Can you work these out from the model? Positions are in its coordinate system, mm. Coordinates: 2 decimals unless noted, no trailing zeros. Loops run counter-clockwise (first coordinate to the right, second up) from the corner with the lowest first, then second, coordinate; pieces in that order, holes last. Notation, with made-up numbers: (-23, 45) -> (11, 45) arc R27 cw to (11, 69) -> close; hole circle Ø6 at (-18.75, 54.25). An arc over 180 degrees is marked (long way). Use one line per item in the form item = value. Start each with the question number.
(1) I need wall thicknesses on line 1 (Z direction, x = -78.5, y = -2.2); line 2 (Z direction, x = -51, y = -2.05); line 3 (X direction, y = -1.1, z = -20). Which ranges of each line are inside material? Lowest first, please. Write a range as [from, to].
(2) Imagine slicing it at B-B (x = -54.5). List the corners of the cut face in (y, z) for me.
(3) Imagine slicing it at A-A (z = -20). List the corners of the cut face in (x, y) for me.
(4) Imagine slicing it at C-C (y = -1.3). List the corners of the cut face in (x, z) for me.
```python
from build123d import *

# Parameters (mm, degrees)
F0_W     = 100
F0_H     = 40
F1_DEPTH = 3
F3_D     = 3
F7_DEPTH = 25
F8_R     = 10


with BuildPart() as f1:
    # F0 (on Front) → F1 (new body)
    with BuildSketch(Plane.XZ):
        with Locations((-50, -20)):
            Rectangle(F0_W, F0_H)
    extrude(amount=F1_DEPTH)

    # F3 (through all)
    with Locations(Plane(origin=(0, 0, 0), x_dir=(1, 0, 0), z_dir=(0, 1, 0))):
        with Locations((-51, 20), (-75, 20)):
            Hole(F3_D / 2)

    # F6 (on face) → F7 (cut)
    with BuildSketch(Plane.XZ.offset(3)):
        with BuildLine():
            ThreePointArc((-80, -27.5), (-82.5, -30), (-80, -32.5))
            Line((-80, -32.5), (-40, -32.5))
            ThreePointArc((-40, -32.5), (-37.5, -30), (-40, -27.5))
            Line((-40, -27.5), (-80, -27.5))
        make_face()
    extrude(amount=-F7_DEPTH, mode=Mode.SUBTRACT)

    # F8
    f8_edges = [f1.edges().sort_by_distance(p)[0] for p in [
        (-100, -1.5, -40),
        (0, -1.5, -40),
    ]]
    fillet(f8_edges, radius=F8_R)

    # F9: F1 across plane


with BuildPart() as f1_1:
    add(f1.part)
    add(f1.part.mirror(Plane.XY))


solid = f1_1.part
```
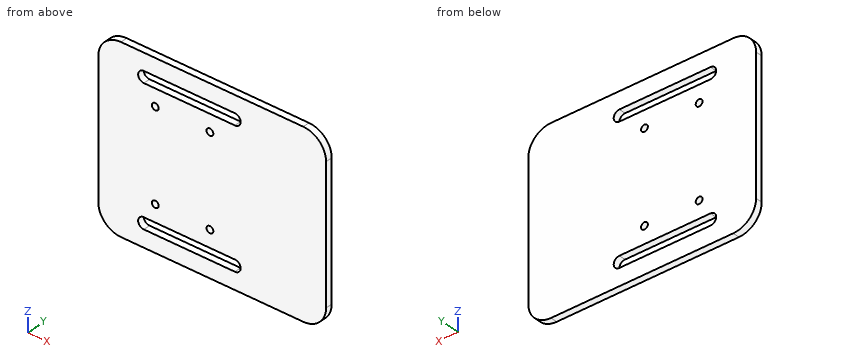
Worked out:
q1.line_1 = [-40, -32.5], [-27.5, 27.5], [32.5, 40]
q1.line_2 = [-40, -32.5], [-27.5, -21.5], [-18.5, 18.5], [21.5, 27.5], [32.5, 40]
q1.line_3 = [-100, -76.5], [-73.5, -52.5], [-49.5, 0]
q2.outline = (-3, -40) -> (0, -40) -> (0, -32.5) -> (-3, -32.5) -> close; (-3, -27.5) -> (0, -27.5) -> (0, 27.5) -> (-3, 27.5) -> close; (-3, 32.5) -> (0, 32.5) -> (0, 40) -> (-3, 40) -> close
q3.outline = (-100, -3) -> (-76.5, -3) -> (-76.5, 0) -> (-100, 0) -> close; (-73.5, -3) -> (-52.5, -3) -> (-52.5, 0) -> (-73.5, 0) -> close; (-49.5, -3) -> (0, -3) -> (0, 0) -> (-49.5, 0) -> close
q4.outline = (-100, -30) arc R10 ccw to (-90, -40) -> (-10, -40) arc R10 ccw to (0, -30) -> (0, 30) arc R10 ccw to (-10, 40) -> (-90, 40) arc R10 ccw to (-100, 30) -> close; hole (-80, -32.5) -> (-40, -32.5) arc R2.5 ccw to (-40, -27.5) -> (-80, -27.5) arc R2.5 ccw to start; hole (-80, 27.5) -> (-40, 27.5) arc R2.5 ccw to (-40, 32.5) -> (-80, 32.5) arc R2.5 ccw to start; hole circle Ø3 at (-75, -20); hole circle Ø3 at (-75, 20); hole circle Ø3 at (-51, -20); hole circle Ø3 at (-51, 20)
